```python
from build123d import *

# Parameters (mm, degrees)
SKETCH_1_R      = 1.3
SKETCH_1_W      = 7.4992
SKETCH_1_H      = 3.0001
SKETCH_1_W_2    = 4.9995
EXTRUDE_1_DEPTH = 3


with BuildPart() as part:
    # 草图1 → 凸台-拉伸1 (new body)
    with BuildSketch(Plane.XY.offset(3)):
        with BuildLine():
            Line((-49.343510787, 0), (30.618171933, 0))
            ThreePointArc((30.618171933, 0), (36.618171933, 6), (30.618171933, 12))
            Line((30.618171933, 12), (-49.343510787, 12))
            ThreePointArc((-49.343510787, 12), (-55.343510787, 6), (-49.343510787, 0))
        make_face()
        with Locations(Location((30.611606698, 6.0001, 0), (0, 0, 180))):
            Circle(SKETCH_1_R, mode=Mode.SUBTRACT)
        with Locations(Location((-1.379286828, 6.00015, 0), (0, 0, 180))):
            Circle(SKETCH_1_R, mode=Mode.SUBTRACT)
        with Locations(Location((-49.343510787, 6, 0), (0, 0, 180))):
            Circle(SKETCH_1_R, mode=Mode.SUBTRACT)
        with Locations((-35.628693302, 5.99945)):
            Rectangle(SKETCH_1_W, SKETCH_1_H, mode=Mode.SUBTRACT)
        with Locations((18.121556698, 5.99945)):
            Rectangle(SKETCH_1_W_2, SKETCH_1_H, mode=Mode.SUBTRACT)
    extrude(amount=-EXTRUDE_1_DEPTH)


solid = part.part
```
Work out the finished part from the listing and answer in its coordinate system (mm). A direction names the side the tool comes from. Give positions to 0.01 mm unless a question says otherwise; leave off trailing zeros. Order: outer loops, then holes, each group sorted by start corner. A loop starts at its lowest first (then second) coordinate and runs counter-clockwise, first axis right, second up. Notation, with made-up numbers: (-8, 83) - (35, 83) arc R17 cw to (35, 99) - close; hole circle Ø11 at (37, 22.5). An arc over 180 degrees is marked (long way). One line per item, written item: value. Start each with the question number.
1. This flat-tipped pin is pushed along its axis until it touches: pin 1 Ø1.5 at (y, z) = (10, 2) entering from +X. Where does it stop, or does it pass through?
2. Which of the six approach directions +Z, -Z, +X, -X, +Y, -Y give full straight-line access (tool end or side, diameter ignored) to faces 1 (the face through (36.617, 5.868, 1.521)), 2 (the face through (-39.378, 6, 2))?
3. Section B-B, the plane y = 9 is taken. Write down the section's boundary in (x, z), then the cut area to 3 significant figures.
4. Consider line 1 (X direction, y = 6, z = 2.4); line 2 (Y direction, x = 18, z = 0.2); line 3 (X direction, y = 5, z = 2.6). Determine where each line is inside the solid, lowest interval first.
5. Section A-A, the plane z = 0.95 is taken. Write down the section's boundary in (x, y).
6. Section C-C, the plane y = 2.75 is taken. Write down the section's boundary in (x, z), then the cut area to 3 significant figures.
7. For a pull along X with two mould halves and no side action, classify faces 3 (the face through (-10, 0, 2)), 4 (the face through (15.622, 6, 2)), 5 (the face through (-55.342, 6.132, 1.521)) as released by +X, released by -X, zero draft, split by the parting line, or undercut.
Filled sheet:
1. pin 1: x = 35.66
2. face 1: +Z, -Z, +X
2. face 2: +Z, -Z
3. outline: (-54.54, 0) - (35.81, 0) - (35.81, 3) - (-54.54, 3) - close
3. area: 271 mm²
4. line 1: -55.34 to -50.64, -48.04 to -39.38, -31.88 to -2.68, -0.08 to 15.62, 20.62 to 29.31, 31.91 to 36.62
4. line 2: 0 to 4.5, 7.5 to 12
4. line 3: -55.26 to -50.17, -48.51 to -39.38, -31.88 to -2.21, -0.55 to 15.62, 20.62 to 29.78, 31.44 to 36.53
5. outline: (-49.34, 0) - (30.62, 0) arc R6 ccw to (30.62, 12) - (-49.34, 12) arc R6 ccw to start; hole circle Ø2.6 at (-49.34, 6); hole (-39.38, 4.5) - (-31.88, 4.5) - (-31.88, 7.5) - (-39.38, 7.5) - close; hole circle Ø2.6 at (-1.38, 6); hole (15.62, 4.5) - (20.62, 4.5) - (20.62, 7.5) - (15.62, 7.5) - close; hole circle Ø2.6 at (30.61, 6)
6. outline: (-54.39, 0) - (35.66, 0) - (35.66, 3) - (-54.39, 3) - close
6. area: 270 mm²
7. face 3: zero draft
7. face 4: undercut
7. face 5: released by -X
